Read the model definition and answer for the solid it produces. Units are mm, in the model's axes. Coordinates: 2 decimals unless noted, no trailing zeros. Write each loop counter-clockwise with the first axis right and the second up, starting at its lowest first coordinate (ties: lowest second). Pieces come first, ordered by that corner, then holes.
(1) The part is cut by section B-B, the plane y = 17. Determine the outline of the cut face in (x, z), and give its area (3 significant figures).
(2) Straight lines are drawn through the part: line 1 along X through (y, z) = (17, 0.95); line 2 along X through (y, z) = (0, 0.2); line 3 along X through (y, z) = (-8, 0.75). For each, find the intervals that lie inside material, in ascending order.
(3) The part is cut by section D-D, the plane z = 1. Determine the outline of the cut face in (x, y), and give its area (3 significant figures).
(4) The part is cut by section C-C, the plane x = 0. Determine the outline of the cut face in (y, z).
(5) The part is cut by section A-A, the plane x = 15.6. Determine the outline of the cut face in (y, z).
(6) Determine the mould class of faces 1 (the flat face through (22.5, 0, 1)), 2 (the flat face through (0, 22.5, 1)), 3 (the cylindrical face through (13.1, -9.1, 1)) for opening direction X: pulls with the +X half, pulls with the -X half, needs draft (parallel to the pull), parting line crosses it, or undercut.
Autodesk Inventor part; units mm, degrees
ref_plane "YZ Plane" through (0, 0, 0) normal (1, 0, 0) x (0, 1, 0)
ref_plane "XZ Plane" through (0, 0, 0) normal (0, 1, 0) x (-1, 0, 0)
ref_plane "XY Plane" through (0, 0, 0) normal (0, 0, 1) x (1, 0, 0)
sketch "Sketch1" plane through (0, 0, 0) normal (0, 0, 1) x (1, 0, 0)
  line L0 (-22.5, -22.5) -> (22.5, -22.5)
  line L1 (22.5, -22.5) -> (22.5, 22.5)
  line L2 (22.5, 22.5) -> (-22.5, 22.5)
  line L3 (-22.5, 22.5) -> (-22.5, -22.5)
  line L4 (-22.5, -22.5) -> (22.5, 22.5) construction
  line L5 (22.5, -22.5) -> (-22.5, 22.5) construction
  circle A0 centre (0, 0) radius 11
  line L6 (0, 0) -> (0, 17)
  line L7 (0, 0) -> (15.6, -9.0067)
  line L8 (0, 0) -> (-15.6, -9.0067)
  circle A1 centre (0, 17) radius 2.5
  circle A2 centre (15.6, -9.0067) radius 2.5
  circle A3 centre (-15.6, -9.0067) radius 2.5
  point P0 (22.5, -11.0947)
  point P1 (-22.5, -11.0947)
  dimension "d0" = 45
  dimension "d1" = 45
  dimension "d2" = 22
  dimension "d3" = 17
  dimension "d4" = 15.6
  dimension "d5" = 120
  dimension "d6" = 15.6
  dimension "d7" = 120
  dimension "d8" = 5
  dimension "d9" = 5
  dimension "d10" = 5
extrude "Extrusion2" add sketch "Sketch1" along normal blind 2
equation "\"d1\" = d0"
equation "\"d4\" = d6"
equation "\"d7\" = d5"
equation "\"d9\" = d8"
equation "\"d10\" = d8"
properties part number "mount_v08"
Computed:
1. outline: (-22.5, 0) - (-2.5, 0) - (-2.5, 2) - (-22.5, 2) - close; (2.5, 0) - (22.5, 0) - (22.5, 2) - (2.5, 2) - close
1. area: 80.0 mm2
2. line 1: x = -22.5 to -2.5, 2.5 to 22.5
2. line 2: x = -22.5 to -11, 11 to 22.5
2. line 3: x = -22.5 to -17.89, -13.31 to -7.55, 7.55 to 13.31, 17.89 to 22.5
3. outline: (-22.5, -22.5) - (22.5, -22.5) - (22.5, 22.5) - (-22.5, 22.5) - close; hole circle Ø5 at (-15.6, -9.01); hole circle Ø22 at (0, 0); hole circle Ø5 at (0, 17); hole circle Ø5 at (15.6, -9.01)
3. area: 1,590 mm2
4. outline: (-22.5, 0) - (-11, 0) - (-11, 2) - (-22.5, 2) - close; (11, 0) - (14.5, 0) - (14.5, 2) - (11, 2) - close; (19.5, 0) - (22.5, 0) - (22.5, 2) - (19.5, 2) - close
5. outline: (-22.5, 0) - (-11.51, 0) - (-11.51, 2) - (-22.5, 2) - close; (-6.51, 0) - (22.5, 0) - (22.5, 2) - (-6.51, 2) - close
6. face 1: pulls with the +X half
6. face 2: needs draft
6. face 3: undercut
